```python
from build123d import *

# Parameters (mm, degrees)
EXTRUDE_THIN1_DEPTH = 15.875
FILLET1_RADIUS      = 7.9375
FILLET1_LENGTH      = 1.6
FILLET2_RADIUS      = 7.9375
FILLET2_LENGTH      = 1.6
SKETCH2_R           = 2.0825
CUT_EXTRUDE1_DEPTH  = 10
SKETCH3_R           = 2.0955
CUT_EXTRUDE2_DEPTH  = 10


with BuildPart() as part:
    # Sketch1 → Extrude-Thin1 (new body)
    with BuildSketch(Plane(origin=(0, 0, 0), x_dir=(1, 0, 0), z_dir=(0, 1, 0))):
        Polygon((0, 20), (0, 0), (-20, 0), (-20, -1.6), (1.6, -1.6), (1.6, 20), align=None)
    extrude(amount=EXTRUDE_THIN1_DEPTH)

    # Fillet1: full round fillet: the end face becomes a half cylinder, R = half its width
    fillet1_face = Plane((0.8, 7.9375, -20), x_dir=(1, 0, 0), z_dir=(0, 0, -1))  # on the end face: x along it, z out of the body
    fillet1_slab = fillet1_face.offset(-FILLET1_RADIUS / 2) * Box(FILLET1_LENGTH, 2 * FILLET1_RADIUS, FILLET1_RADIUS, mode=Mode.PRIVATE)  # the body's end, R deep
    fillet1_round = Plane((0.8, 7.9375, -12.0625), x_dir=(0, 0, -1), z_dir=(1, 0, 0)) * Cylinder(FILLET1_RADIUS, FILLET1_LENGTH, mode=Mode.PRIVATE)  # its axis R under the face
    add(fillet1_slab - fillet1_round, mode=Mode.SUBTRACT)

    # Fillet2: full round fillet: the end face becomes a half cylinder, R = half its width
    fillet2_face = Plane((-20, 7.9375, 0.8), x_dir=(0, 0, 1), z_dir=(-1, 0, 0))  # on the end face: x along it, z out of the body
    fillet2_slab = fillet2_face.offset(-FILLET2_RADIUS / 2) * Box(FILLET2_LENGTH, 2 * FILLET2_RADIUS, FILLET2_RADIUS, mode=Mode.PRIVATE)  # the body's end, R deep
    fillet2_round = Plane((-12.0625, 7.9375, 0.8), x_dir=(-1, 0, 0), z_dir=(0, 0, 1)) * Cylinder(FILLET2_RADIUS, FILLET2_LENGTH, mode=Mode.PRIVATE)  # its axis R under the face
    add(fillet2_slab - fillet2_round, mode=Mode.SUBTRACT)

    # Sketch2 → Cut-Extrude1 (cut)
    with BuildSketch(Plane.ZY):
        with Locations((-12.0625, 7.9375)):
            Circle(SKETCH2_R)
    extrude(amount=-CUT_EXTRUDE1_DEPTH, mode=Mode.SUBTRACT)

    # Sketch3 → Cut-Extrude2 (cut)
    with BuildSketch(Plane(origin=(0, 0, 0), x_dir=(-1, 0, 0), z_dir=(0, 0, -1))):
        with Locations((12.0625, 7.9375)):
            Circle(SKETCH3_R)
    extrude(amount=-CUT_EXTRUDE2_DEPTH, mode=Mode.SUBTRACT)


solid = part.part
```
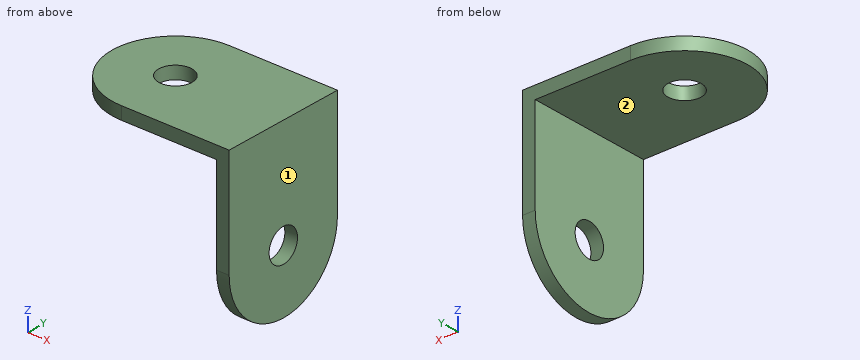
The listing builds one solid part. Answer for the finished solid, in the listing's coordinates (mm). Face numbers are marked on the shaded views. A direction names the side the tool comes from. Round coordinates to 2 decimals unless told otherwise and drop trailing zeros. Loops run counter-clockwise (first coordinate to the right, second up) from the corner with the lowest first, then second, coordinate; pieces in that order, holes last.
Q1. Section C-C, the plane x = -13.5 is taken. Determine the outline of the cut face in (y, z), then the cut area to 3 significant figures.
Q2. Section B-B, the plane z = -13 is taken. Determine the outline of the cut face in (x, y), then the cut area to 3 significant figures.
Q3. Find the intervals of material crossed by line 1 (X direction, y = 1, z = -13.75); line 2 (Y direction, x = -16.5, z = 0.5), in increasing order.
Q4. Section A-A, the plane y = 7 is taken. Determine the outline of the cut face in (x, z), then the cut area to 3 significant figures.
Q5. Section D-D, the plane y = 9 is taken. Determine the outline of the cut face in (x, z).
Q6. Which of the six approach directions +Z, -Z, +X, -X, +Y, -Y give full straight-line access (tool end or side, diameter ignored) to the marked faces 1 and 2?
Q7. Given pin 1 Ø2.5 at (x, y) = (-12.06, 7.94) entering from -Z; pin 2 Ø1 at (y, z) = (5.5, -6) entering from -X; pin 3 Ø8 at (x, y) = (-16, 3.5) entering from -Z, each flat-ended and moving along its own axis, determine where each tip first touches the part or whether it passes through.
Completed:
1. outline: (0.13, 0) - (6.41, 0) - (6.41, 1.6) - (0.13, 1.6) - close; (9.46, 0) - (15.74, 0) - (15.74, 1.6) - (9.46, 1.6) - close
1. area: 20.1 mm2
2. outline: (0, 0.06) - (1.6, 0.06) - (1.6, 6.08) - (0, 6.08) - close; (0, 9.8) - (1.6, 9.8) - (1.6, 15.82) - (0, 15.82) - close
2. area: 19.3 mm2
3. line 1: x = 0 to 1.6
3. line 2: y = 1.36 to 14.52
4. outline: (-19.94, 0) - (-13.94, 0) - (-13.94, 1.6) - (-19.94, 1.6) - close; (-10.19, 0) - (0, 0) - (0, -10.2) - (1.6, -10.2) - (1.6, 1.6) - (-10.19, 1.6) - close; (0, -19.94) - (1.6, -19.94) - (1.6, -13.92) - (0, -13.92) - close
4. area: 54.4 mm2
5. outline: (-19.93, 0) - (-13.87, 0) - (-13.87, 1.6) - (-19.93, 1.6) - close; (-10.26, 0) - (0, 0) - (0, -10.27) - (1.6, -10.27) - (1.6, 1.6) - (-10.26, 1.6) - close; (0, -19.93) - (1.6, -19.93) - (1.6, -13.85) - (0, -13.85) - close
6. face 1: +Z, -Z, +X, +Y, -Y
6. face 2: -Z, -X, +Y, -Y
7. pin 1: passes through
7. pin 2: stops at x = 0
7. pin 3: stops at z = 0
